Geometry: final body of the model. Coordinates: model frame, mm. A direction names the side the tool comes from. Round coordinates to 2 decimals unless told otherwise and drop trailing zeros. Write each loop counter-clockwise with the first axis right and the second up, starting at its lowest first coordinate (ties: lowest second). Pieces come first, ordered by that corner, then holes. Notation, with made-up numbers: M -23.75,11 L 34.25,11 A21 cw 34.25,48 Z; hole C 3.5,22.5 d4. An arc over 180 degrees is marked long. Use one line per item in the form item = value. Start each with the question number.
Item 1: Reachability of faces 1 (the flat face through (61, 211, 0)), 2 (the flat face through (30, 233, 0)), 3 (the flat face through (5, 221, -16)), 4 (the flat face through (29, 206, -36)) from +Z, -Z, +X, -X, +Y, -Y: full face, straight path, thin tool, end or side. Return the list, or none.
Item 2: Pin query (flat end, axial travel): pin 1 Ø1.8 at (y, z) = (186, -4) entering from +X; pin 2 Ø1 at (x, y) = (37, 208) entering from +Z; pin 3 Ø9.5 at (x, y) = (14.5, 199.5) entering from +Z. Return the tip coordinate at first contact, or that it passes through.
Item 3: Section query A-A (z = -0.5). Return loops of the section in (x, y), and give its area (3 significant figures).
Item 4: Ray query, probe 1 along X at (y, z) = (204, -12); probe 2 along Y at (x, z) = (39, -28); probe 3 along Y at (x, z) = (18.5, 1). Return the intervals inside material, ascending.
Item 5: Pull-direction query (X, two-part tool) for faces 5 (the flat face through (66, 206, -19)), 6 (the flat face through (29, 174, -19)), 7 (the flat face through (15, 228, 2)); classes: pulls with the +X half, pulls with the -X half, needs draft (parallel to the pull), parting line crosses it, or undercut.
Item 6: Section query D-D (z = -13.5). Return loops of the section in (x, y).
Item 7: Section query B-B (y = 208). Return loops of the section in (x, z).
from build123d import *

# Parameters (mm, degrees)
BOX011_W        = 60
BOX011_H        = 11
BOX011_DEPTH    = 1.9
BOX010_W        = 72
BOX010_H        = 8
BOX010_DEPTH    = 34
BOX009_W        = 6
BOX009_H        = 49
BOX009_DEPTH    = 34
BOX008_W        = 6
BOX008_H        = 64
BOX008_DEPTH    = 34
BOX007_W        = 72
BOX007_H        = 6
BOX007_DEPTH    = 34
BOX003_W        = 25
BOX003_H        = 16
BOX003_DEPTH    = 4
CHAMFER001_SIZE = 3
BOX002_W        = 21
BOX002_H        = 12
BOX002_DEPTH    = 35
BOX004_W        = 62
BOX004_H        = 44
BOX004_DEPTH    = 39
BOX012_W        = 72
BOX012_H        = 15
BOX012_DEPTH    = 28


with BuildPart() as cube010:
    # Box011 → Box011 (new body)
    with BuildSketch(Plane(origin=(6, 179, -7.5), x_dir=(1, 0, 0), z_dir=(0, 0, 1))):
        with Locations((30, 5.5)):
            Rectangle(BOX011_W, BOX011_H)
    extrude(amount=BOX011_DEPTH)


with BuildPart() as cube009:
    # Box010 → Box010 (new body)
    with BuildSketch(Plane(origin=(-6, 230, -36), x_dir=(1, 0, 0), z_dir=(0, 0, 1))):
        with Locations((36, 4)):
            Rectangle(BOX010_W, BOX010_H)
    extrude(amount=BOX010_DEPTH)


with BuildPart() as cube008:
    # Box009 → Box009 (new body)
    with BuildSketch(Plane(origin=(60, 189, -36), x_dir=(1, 0, 0), z_dir=(0, 0, 1))):
        with Locations((3, 24.5)):
            Rectangle(BOX009_W, BOX009_H)
    extrude(amount=BOX009_DEPTH)


with BuildPart() as cube007:
    # Box008 → Box008 (new body)
    with BuildSketch(Plane(origin=(-6, 174, -36), x_dir=(1, 0, 0), z_dir=(0, 0, 1))):
        with Locations((3, 32)):
            Rectangle(BOX008_W, BOX008_H)
    extrude(amount=BOX008_DEPTH)


with BuildPart() as cube006:
    # Box007 → Box007 (new body)
    with BuildSketch(Plane(origin=(-6, 174, -36), x_dir=(1, 0, 0), z_dir=(0, 0, 1))):
        with Locations((36, 3)):
            Rectangle(BOX007_W, BOX007_H)
    extrude(amount=BOX007_DEPTH)


with BuildPart() as chamfer001:
    # Box003 → Box003 (new body)
    with BuildSketch(Plane(origin=(-2, -2, 32), x_dir=(1, 0, 0), z_dir=(0, 0, 1))):
        with Locations((12.5, 8)):
            Rectangle(BOX003_W, BOX003_H)
    extrude(amount=BOX003_DEPTH)

    # Chamfer001
    chamfer001_edges = [chamfer001.edges().sort_by_distance(p)[0] for p in [
        (-2, 6, 32),
        (23, 6, 32),
        (10.5, -2, 32),
        (10.5, 14, 32),
    ]]
    chamfer(chamfer001_edges, length=CHAMFER001_SIZE)


with BuildPart() as obj1:
    # Box002 → Box002 (new body)
    with BuildSketch(Plane.XY):
        with Locations((10.5, 6)):
            Rectangle(BOX002_W, BOX002_H)
    extrude(amount=BOX002_DEPTH)

    # Fusion001: union Chamfer001
    add(chamfer001.part)


with BuildPart() as obj1_1:
    # Fusion001 placement: moved
    add(obj1.part.moved(Location((30, 175, 0))))


with BuildPart() as obj2:
    # Clone001 base: copy of obj1
    add(obj1_1.part)


with BuildPart() as obj2_1:
    # Clone001 placement: moved
    add(obj2.part.moved(Location((-30, 0, 0))))


with BuildPart() as obj3:
    # Clone base: copy of obj1
    add(obj1_1.part)


with BuildPart() as obj3_1:
    # Clone placement: moved
    add(obj3.part.moved(Location((0, -20, 0))))


with BuildPart() as obj4:
    # Clone002 base: copy of obj1
    add(obj1_1.part)


with BuildPart() as obj4_1:
    # Clone002 placement: moved
    add(obj4.part.moved(Location((-30, -20, 0))))

    # Fusion002: union obj1, obj2, obj3
    add(obj1_1.part)
    add(obj2_1.part)
    add(obj3_1.part)


with BuildPart() as obj4_2:
    # Fusion002 placement: moved
    add(obj4_1.part.moved(Location((5, 0, 4))))


with BuildPart() as usbhalter:
    # Box004 → Box004 (new body)
    with BuildSketch(Plane(origin=(-1, 149, 0), x_dir=(1, 0, 0), z_dir=(0, 0, 1))):
        with Locations((31, 22)):
            Rectangle(BOX004_W, BOX004_H)
    extrude(amount=BOX004_DEPTH)

    # Cut: cut obj4
    add(obj4_2.part, mode=Mode.SUBTRACT)


with BuildPart() as usbhalter_1:
    # Cut placement: moved
    add(usbhalter.part.moved(Location((0, 40, -36))))


with BuildPart() as halterblock:
    # Box012 → Box012 (new body)
    with BuildSketch(Plane(origin=(-6, 174, -36), x_dir=(1, 0, 0), z_dir=(0, 0, 1))):
        with Locations((36, 7.5)):
            Rectangle(BOX012_W, BOX012_H)
    extrude(amount=BOX012_DEPTH)

    # Fusion003: union Cube009, Cube008, Cube007, Cube006, USBHalter
    add(cube009.part)
    add(cube008.part)
    add(cube007.part)
    add(cube006.part)
    add(usbhalter_1.part)

    # Cut003: cut Cube010
    add(cube010.part, mode=Mode.SUBTRACT)


solid = halterblock.part
Working result:
q1.face_1 = +Z, +X, +Y, -Y
q1.face_2 = +Z, +X, -X, +Y
q1.face_3 = +Z
q1.face_4 = -Z, +X, -X, +Y, -Y
q2.pin_1 = 0
q2.pin_2 = 2.5
q2.pin_3 = 1.25
q3.outline = M -1,189 L 61,189 L 61,233 L -1,233 Z; hole M 5,195 L 26,195 L 26,207 L 5,207 Z; hole M 5,215 L 26,215 L 26,227 L 5,227 Z; hole M 35,195 L 56,195 L 56,207 L 35,207 Z; hole M 35,215 L 56,215 L 56,227 L 35,227 Z
q3.area = 1,720 mm²
q4.probe_1 = -6 to 5, 26 to 35, 56 to 66
q4.probe_2 = 174 to 195, 207 to 215, 227 to 238
q4.probe_3 = 189 to 195, 207 to 215, 227 to 233
q5.face_5 = pulls with the +X half
q5.face_6 = needs draft
q5.face_7 = undercut
q6.outline = M -6,174 L 66,174 L 66,238 L -6,238 Z; hole M 5,195 L 26,195 L 26,207 L 5,207 Z; hole M 5,215 L 26,215 L 26,227 L 5,227 Z; hole M 35,195 L 56,195 L 56,207 L 35,207 Z; hole M 35,215 L 56,215 L 56,227 L 35,227 Z
q7.outline = M -6,-36 L 66,-36 L 66,-2 L 61,-2 L 61,3 L 58,3 L 57,2 L 34,2 L 33,3 L 28,3 L 27,2 L 4,2 L 3,3 L -1,3 L -1,-2 L -6,-2 Z
